Verification items for the finished model (mm, model axes). Face numbers are marked on the shaded views. Round coordinates to 2 decimals unless told otherwise and drop trailing zeros. Loops run counter-clockwise (first coordinate to the right, second up) from the corner with the lowest first, then second, coordinate; pieces in that order, holes last. Notation, with made-up numbers: (72.5, 8) -> (93.5, 8) arc R25 ccw to (93.5, 41) -> close; hole circle Ø10 at (20, 56.25). An arc over 180 degrees is marked (long way). Write item = value, one per line.
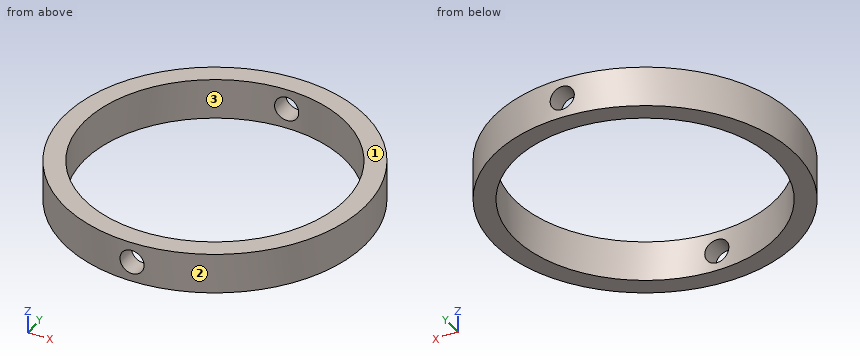
```python
from build123d import *

# Parameters (mm, degrees)
SKETCH1_R               = 47.625
SKETCH1_R_2             = 41.275
BOSS_EXTRUDE1_DEPTH     = 12.7
CUT_EXTRUDE1_REACH      = 109.247
CUT_EXTRUDE1_END_RADIUS = 41.275
SKETCH2_R               = 3.81


with BuildPart() as part:
    # Sketch1 → Boss-Extrude1 (new body)
    with BuildSketch(Plane.XY):
        Circle(SKETCH1_R)
        Circle(SKETCH1_R_2, mode=Mode.SUBTRACT)
    extrude(amount=BOSS_EXTRUDE1_DEPTH)

    # Cut-Extrude1: up to this cylinder (the profile starts outside it)
    cut_extrude1_end = Plane(origin=(0, 0, 6.35), z_dir=(0, 0, -1)) * Cylinder(CUT_EXTRUDE1_END_RADIUS, 302.044, mode=Mode.PRIVATE)
    # Sketch2 → Cut-Extrude1 (cut, up to the surface)
    with BuildSketch(Plane(origin=(0, 47.625, 0), x_dir=(1, 0, 0), z_dir=(0, 1, 0)), mode=Mode.PRIVATE) as cut_extrude1_sk1:
        with Locations(Location((0, -6.35, 0), (0, 0, 270))):
            Circle(SKETCH2_R)
    cut_extrude1_tool1 = extrude(cut_extrude1_sk1.sketch, amount=-CUT_EXTRUDE1_REACH, mode=Mode.PRIVATE) - cut_extrude1_end
    cut_extrude1 = cut_extrude1_tool1.solids().sort_by_distance((0, 47.625, 6.35))[0]
    add(cut_extrude1, mode=Mode.SUBTRACT)

    # Mirror1: Cut-Extrude1 across plane
    add(cut_extrude1.mirror(Plane.ZX), mode=Mode.SUBTRACT)


solid = part.part
```
(1) Go/stop test with flat-tipped pins: pin 1 Ø6 at (x, z) = (-35, 3) entering from -Y; pin 2 Ø4 at (y, z) = (-17.5, 11) entering from -X; pin 3 Ø5 at (x, z) = (26, 1.5) entering from +Y. Record where each tip stops, or that it passes through.
Filled sheet:
pin_1 = -35.27
pin_2 = -45.03
pin_3 = 41.42
(2) Draft check along X on the marked faces 1, 2 and 3. Enter one of: released by +X, released by -X, zero draft, split by the parting line, or undercut.
Filled sheet:
face_1 = zero draft
face_2 = split by the parting line
face_3 = undercut
(3) Material ranges on probe 1 along Z at (x, y) = (0, 43); probe 2 along X at (y, z) = (-8, 1); probe 3 along X at (y, z) = (-34, 1.5), recorded low to high. Write a range as from..to.
Filled sheet:
probe_1 = 0..2.54, 10.16..12.7
probe_2 = -46.95..-40.49, 40.49..46.95
probe_3 = -33.35..-23.4, 23.4..33.35
(4) Sectioned sample at C-C, the plane z = 7.25. Record the cut outline in (x, y) (3 decimals).
Filled sheet:
outline = (-3.702, -47.481) -> (-3.702, -41.109) arc R41.275 cw to (-3.702, 41.109) -> (-3.702, 47.481) arc R47.625 ccw to start; (3.702, -47.481) arc R47.625 ccw to (3.702, 47.481) -> (3.702, 41.109) arc R41.275 cw to (3.702, -41.109) -> close
(5) Sectioned sample at B-B, the plane x = 0. Record the cut outline in (y, z) (3 decimals).
Filled sheet:
outline = (-47.625, 0) -> (-41.275, 0) -> (-41.275, 2.54) -> (-47.625, 2.54) -> close; (-47.625, 10.16) -> (-41.275, 10.16) -> (-41.275, 12.7) -> (-47.625, 12.7) -> close; (41.275, 0) -> (47.625, 0) -> (47.625, 2.54) -> (41.275, 2.54) -> close; (41.275, 10.16) -> (47.625, 10.16) -> (47.625, 12.7) -> (41.275, 12.7) -> close
(6) Sectioned sample at A-A, the plane y = 0. Record the cut outline in (x, z) (3 decimals).
Filled sheet:
outline = (-47.625, 0) -> (-41.275, 0) -> (-41.275, 12.7) -> (-47.625, 12.7) -> close; (41.275, 0) -> (47.625, 0) -> (47.625, 12.7) -> (41.275, 12.7) -> close
